```python
from build123d import *

# Parameters (mm, degrees)
SKETCH_1_R          = 1.25
SKETCH_1_R_2        = 0.5
EXTRUDE_1_DEPTH     = 2
CUT_EXTRUDE_1_REACH = 17.532
SKETCH_2_R          = 0.5
EXTRUDE_START       = 2.5
SKETCH_3_R          = 3.5
SKETCH_3_R_2        = 2.5
EXTRUDE_2_DEPTH     = 2.5


with BuildPart() as part:
    # 草圖1 → 填料-伸長1 (new body)
    with BuildSketch(Plane.XY):
        with BuildLine():
            Line((0, 3.5), (13.227281041, 1.987043867))
            ThreePointArc((13.227281041, 1.987043867), (14.99675834, -0.113825012), (13, -2))
            Line((13, -2), (0, -3.5))
            ThreePointArc((0, -3.5), (-3.5, 0), (0, 3.5))
        make_face()
        Circle(SKETCH_1_R, mode=Mode.SUBTRACT)
        with Locations((13, 0)):
            Circle(SKETCH_1_R_2, mode=Mode.SUBTRACT)
    extrude(amount=EXTRUDE_1_DEPTH)

    # 草圖2 → 除料-伸長1 (cut, up to next)
    with BuildSketch(Plane.XY.offset(2), mode=Mode.PRIVATE) as cut_extrude_1_sk1:
        with Locations((10.5, 0)):
            Circle(SKETCH_2_R)
    cut_extrude_1_tool1 = extrude(cut_extrude_1_sk1.sketch, amount=-CUT_EXTRUDE_1_REACH, mode=Mode.PRIVATE) & part.part
    # 草圖2 → 除料-伸長1 (cut, up to next)
    with BuildSketch(Plane.XY.offset(2), mode=Mode.PRIVATE) as cut_extrude_1_sk2:
        with Locations((8, 0)):
            Circle(SKETCH_2_R)
    cut_extrude_1_tool2 = extrude(cut_extrude_1_sk2.sketch, amount=-CUT_EXTRUDE_1_REACH, mode=Mode.PRIVATE) & part.part
    # 草圖2 → 除料-伸長1 (cut, up to next)
    with BuildSketch(Plane.XY.offset(2), mode=Mode.PRIVATE) as cut_extrude_1_sk3:
        with Locations((5, 0)):
            Circle(SKETCH_2_R)
    cut_extrude_1_tool3 = extrude(cut_extrude_1_sk3.sketch, amount=-CUT_EXTRUDE_1_REACH, mode=Mode.PRIVATE) & part.part
    add(cut_extrude_1_tool1.solids().sort_by_distance((10.5, 0, 2))[0], mode=Mode.SUBTRACT)
    add(cut_extrude_1_tool2.solids().sort_by_distance((8, 0, 2))[0], mode=Mode.SUBTRACT)
    add(cut_extrude_1_tool3.solids().sort_by_distance((5, 0, 2))[0], mode=Mode.SUBTRACT)

    # 草圖3 → 填料-伸長2 (add)
    with BuildSketch(Plane(origin=(0, 0, 0), x_dir=(-1, 0, 0), z_dir=(0, 0, -1)).offset(EXTRUDE_START)):
        Circle(SKETCH_3_R)
        Circle(SKETCH_3_R_2, mode=Mode.SUBTRACT)
    extrude(amount=-EXTRUDE_2_DEPTH)


solid = part.part
```
Read the model definition and answer for the solid it produces. Units are mm, in the model's axes. A direction names the side the tool comes from. Give positions to 0.01 mm unless a question says otherwise; leave off trailing zeros. Write each loop counter-clockwise with the first axis right and the second up, starting at its lowest first coordinate (ties: lowest second). Pieces come first, ordered by that corner, then holes. Notation, with made-up numbers: (-28.5, 50) - (8.5, 50) arc R20 cw to (8.5, 87) - close; hole circle Ø6 at (26, 87.5). An arc over 180 degrees is marked (long way). Write item = value, one per line. Start each with the question number.
Item 1: Find section D-D (z = -1). Give the vertices of the cut face in (x, y), then the cut area to 3 significant figures.
Item 2: The mould has two halves that part along Y. Classify faces 1 (the flat face through (6.521, 2.754, 0.986)), 2 (the cylindrical face through (-3.086, -1.651, 0.219)), 3 (the cylindrical face through (10, 0, 1)), 4 (the cylindrical face through (8.462, -0.192, 1.014)): +Y half, -Y half, draft (parallel to the pull), parting line (faces both ways), or undercut.
Item 3: Find section B-B (x = 10.5). Give the vertices of the cut face in (y, z).
Item 4: Find section A-A (z = 0.3). Give the vertices of the cut face in (x, y), then the cut area to 3 significant figures.
Item 5: Find section C-C (x = 3). Give the vertices of the cut face in (y, z).
Item 6: A tool of negligible diameter and unlimited length cuts with its end or side. For faces 5 (the cylindrical face through (12.5, 0, 1)), 6 (the flat face through (-1, 1, 0)), from which of +Z, -Z, +X, -X, +Y, -Y can it reach the whole face along a straight path? Write none if from no direction.
Item 7: Find the intervals of material crossed by probe 1 along Y at (x, z) = (0, 0.7); probe 2 along Y at (x, z) = (0, -0.55); probe 3 along Z at (x, y) = (4, -0.25), in increasing order. Write a range as [from, to].
Response:
q1.outline = circle Ø7 at (0, 0); hole circle Ø5 at (0, 0)
q1.area = 18.8 mm²
q2.face_1 = +Y half
q2.face_2 = parting line
q2.face_3 = undercut
q2.face_4 = undercut
q3.outline = (-2.29, 0) - (-0.5, 0) - (-0.5, 2) - (-2.29, 2) - close; (0.5, 0) - (2.3, 0) - (2.3, 2) - (0.5, 2) - close
q4.outline = (0, -3.5) - (13, -2) arc R2 ccw to (13.23, 1.99) - (0, 3.5) arc R3.5 ccw to start; hole circle Ø2.5 at (0, 0); hole circle Ø1 at (5, 0); hole circle Ø1 at (8, 0); hole circle Ø1 at (10.5, 0); hole circle Ø1 at (13, 0)
q4.area = 89.1 mm²
q5.outline = (-3.15, 0) - (-1.8, 0) - (-1.8, -2.5) - (1.8, -2.5) - (1.8, 0) - (3.16, 0) - (3.16, 2) - (-3.15, 2) - close
q6.face_5 = +Z, -Z
q6.face_6 = -Z
q7.probe_1 = [-3.5, -1.25], [1.25, 3.5]
q7.probe_2 = [-3.5, -2.5], [2.5, 3.5]
q7.probe_3 = [0, 2]
